```python
from build123d import *

# Parameters (mm, degrees)
SKETCH1_R     = 2.5
BASE_DEPTH    = 8.6
DOME_R        = 2.5
BASECUT_DEPTH = 1


with BuildPart() as part:
    # Sketch1 → Base (new body)
    with BuildSketch(Plane(origin=(0, 0, 0), x_dir=(1, 0, 0), z_dir=(0, 1, 0))):
        with Locations(Location((0, 0, 0), (0, 0, 90))):
            Circle(SKETCH1_R)
    extrude(amount=BASE_DEPTH)

    # Dome
    dome_edges = [part.edges().sort_by_distance(p)[0] for p in [
        (0, 8.6, 2.5),
    ]]
    fillet(dome_edges, radius=DOME_R)

    # BaseCutSketch → BaseCut (add)
    with BuildSketch(Plane(origin=(0, 0, 0), x_dir=(1, 0, 0), z_dir=(0, 1, 0))):
        with BuildLine():
            Line((1.566045976, -2.5), (-1.566045976, -2.5))
            ThreePointArc((-1.566045976, -2.5), (0, 2.95), (1.566045976, -2.5))
        make_face()
    extrude(amount=BASECUT_DEPTH)


solid = part.part
```
The model under review builds one solid part; all positions refer to its coordinate system, in mm. A direction names the side the tool comes from. Round coordinates to 2 decimals unless told otherwise and drop trailing zeros. Loops run counter-clockwise (first coordinate to the right, second up) from the corner with the lowest first, then second, coordinate; pieces in that order, holes last. Notation, with made-up numbers: M 85.25,7 L 134.25,7 A19 ccw 134.25,42 Z; hole C 70,-34.5 d4. An arc over 180 degrees is marked long. Put each result on its own line as item: value.
Q1. Consider section A-A, the plane z = 0. Give the boundary of the cut face in (x, y).
Result set:
outline: M -2.95,0 L 2.95,0 L 2.95,1 L 2.5,1 L 2.5,6.1 A2.5 ccw -2.5,6.1 L -2.5,1 L -2.95,1 Z
Q2. For pin 1 (2 mm diameter, centred on x = -2, z = 0.5, fed in from +Y); pin 2 (3 mm diameter, centred on y = 4, z = 1, fed in from +X); pin 3 (2 mm diameter, centred on x = 1, y = 1.5, fed in from -Z), all flat-tipped, find the tip position at first contact; note any pin that passes through.
Result set:
pin 1: stops at y = 8.36
pin 2: stops at x = 2.5
pin 3: stops at z = -2.95
Q3. To check wall thickness, follow L1, parallel to Y at x = -2.5, z = -0.7; L2, parallel to Z at x = 1.2, y = 4.75; L3, parallel to Y at x = 1.5, z = -0.15. State the ranges of each line that lie inside material, in increasing order.
Result set:
L1: y = 0 to 1
L2: z = -2.19 to 2.19
L3: y = 0 to 8.09
Q4. Consider section B-B, the plane x = -1.9. Give the boundary of the cut face in (y, z).
Result set:
outline: M 0,-2.26 L 1,-2.26 L 1,-1.62 L 6.1,-1.62 A1.62 ccw 6.1,1.62 L 1,1.62 L 1,2.26 L 0,2.26 Z
Q5. Consider section C-C, the plane y = 2. Give the boundary of the cut face in (x, z).
Result set:
outline: C 0,0 d5
Q6. Consider section D-D, the plane y = 6.25. Give the boundary of the cut face in (x, z), then the cut area to 3 significant figures.
Result set:
outline: C 0,0 d4.99
area: 19.6 mm²
Q7. Machinability: for faces 1 (the cylindrical face through (-0.107, 0.493, -2.948)), 2 (the flat face through (0.9, 1, -2.5)), which of the approach directions +Z, -Z, +X, -X, +Y, -Y give a long, thin tool a straight path to every point of the face, cutting with its end or side? Answer none if there is none.
Result set:
face 1: +Y, -Y
face 2: +Y
